The figure shows three views and two pictorial views of one solid part (mm, origin at its lowest corner). Answer the questions. A direction names the side the tool comes from. Round coordinates to 2 decimals unless told otherwise and drop trailing zeros. Order: outer loops, then holes, each group sorted by start corner. A loop starts at its lowest first (then second) coordinate and runs counter-clockwise, first axis right, second up. Notation, with made-up numbers: (-17.75, 64.25) - (-2.75, 64.25) arc R22 cw to (-2.75, 85.25) - close; hole circle Ø3 at (80.25, -19.75). An arc over 180 degrees is marked (long way). One line per question, with ' | ' between items. Start each with the question number.
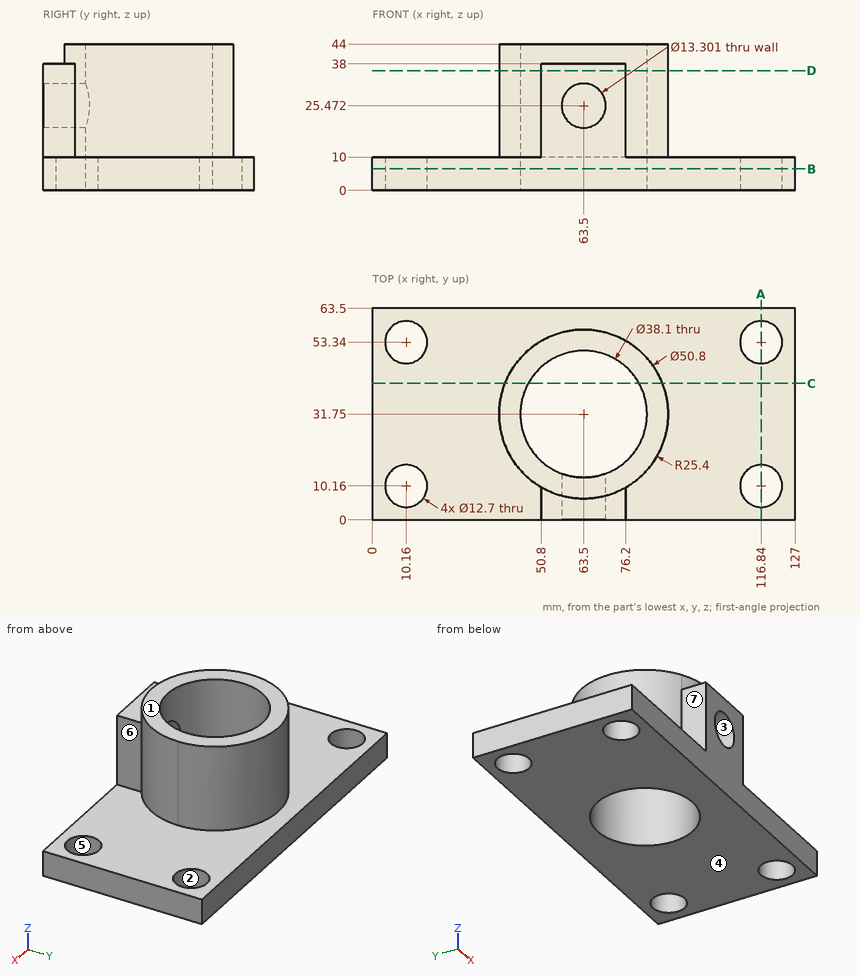
1) Section D-D on z = 36 is taken. Give the vertices of the cut face in (x, y), and give its area (3 significant figures).
2) Straight lines are drawn through the part: line 1 (Y direction, x = 116.84, z = 6.25); line 2 (X direction, y = 53, z = 3); line 3 (X direction, y = 31, z = 27) (1 decimal). For each, find the intervals that lie inside material, in ascending order.
3) Section B-B on z = 6.5 is taken. Give the vertices of the cut face in (x, y), and give its area (3 significant figures).
4) Section A-A on x = 116.84 is taken. Give the vertices of the cut face in (y, z), and give its area (3 significant figures).
5) Flat-ended cylindrical pins translate along their axes: pin 1 (2 mm diameter, centred on x = 60.5, z = 22, fed in from -Y) (1 decimal); pin 2 (10.5 mm diameter, centred on x = 63.5, z = 25.47, fed in from +Y); pin 3 (14.5 mm diameter, centred on x = 10.16, y = 53.34, fed in from +Z). Find the tip coordinate at first contact, or state that the pin passes through.
6) Determine the mould class of the marked faces 1, 2, 3 and 4 for opening direction Z: released by +Z, released by -Z, zero draft, split by the parting line, or undercut.
7) Section C-C on y = 41 is taken. Give the vertices of the cut face in (x, z).
8) For the marked faces 5, 6 and 7, determine the directions among +Z, -Z, +X, -X, +Y, -Y from which every point of the face is accessible in a straight line to the end or side of a thin tool.
Recorded:
1) outline: (50.8, 0) - (76.2, 0) - (76.2, 9.75) arc R25.4 ccw (long way) to (50.8, 9.75) - close; hole circle Ø38.1 at (63.5, 31.75) | area: 1,080 mm²
2) line 1: y = 0 to 3.81, 16.51 to 46.99, 59.69 to 63.5 | line 2: x = 0 to 3.82, 16.5 to 110.5, 123.18 to 127 | line 3: x = 38.1 to 44.5, 82.5 to 88.9
3) outline: (0, 0) - (127, 0) - (127, 63.5) - (0, 63.5) - close; hole circle Ø12.7 at (10.16, 10.16); hole circle Ø12.7 at (10.16, 53.34); hole circle Ø38.1 at (63.5, 31.75); hole circle Ø12.7 at (116.84, 10.16); hole circle Ø12.7 at (116.84, 53.34) | area: 6,420 mm²
4) outline: (0, 0) - (3.81, 0) - (3.81, 10) - (0, 10) - close; (16.51, 0) - (46.99, 0) - (46.99, 10) - (16.51, 10) - close; (59.69, 0) - (63.5, 0) - (63.5, 10) - (59.69, 10) - close | area: 381 mm²
5) pin 1: stops at y = 50.4 | pin 2: stops at y = 57.15 | pin 3: stops at z = 10
6) face 1: released by +Z | face 2: zero draft | face 3: undercut | face 4: released by -Z
7) outline: (0, 0) - (46.85, 0) - (46.85, 44) - (39.84, 44) - (39.84, 10) - (0, 10) - close; (80.15, 0) - (127, 0) - (127, 10) - (87.16, 10) - (87.16, 44) - (80.15, 44) - close
8) face 5: +Z, -Z | face 6: +Z, +X, -Y | face 7: +Z, -X, -Y
